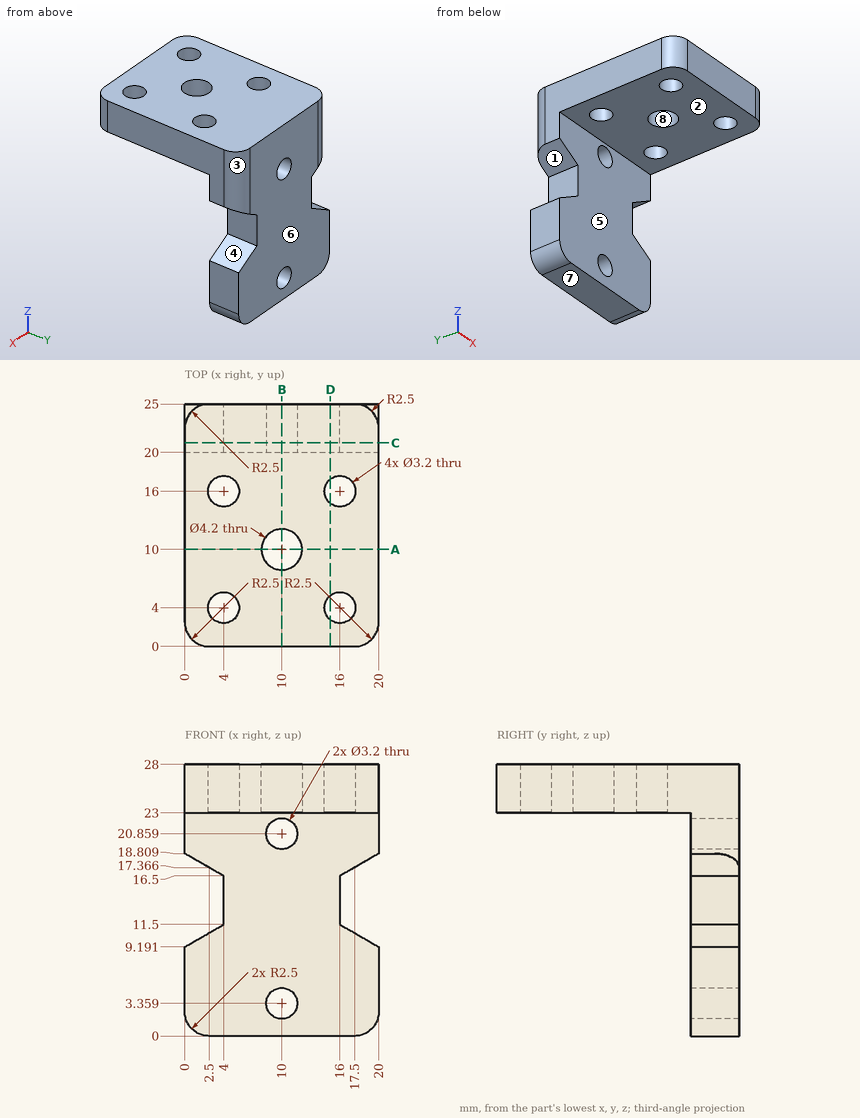
Can you work these out from the drawing? Everything is in mm from the part's minimum corner. A direction names the side the tool comes from. Coordinates: 2 decimals unless noted, no trailing zeros. Loops run counter-clockwise (first coordinate to the right, second up) from the corner with the lowest first, then second, coordinate; pieces in that order, holes last.
1. Imagine slicing it at D-D, the plane x = 15. Please give me the cut outline in (y, z), and give its area (3 significant figures).
2. For the marked faces 1, 2, 3 and 4, which set-ups out of +Z, -Z, +X, -X, +Y, -Y let a thin tool reach every point of the face, with its end or its side?
3. Imagine slicing it at A-A, the plane y = 10. Please give me the cut outline in (x, z).
4. Imagine slicing it at B-B, the plane x = 10. Please give me the cut outline in (y, z).
5. I need wall thicknesses on L1, parallel to Y at x = 4, z = 24.7; L2, parallel to Z at x = 10.5, y = 21.25; L3, parallel to Y at x = 1.75, z = 5.5. Which ranges of each line are inside material? Lowest first, please.
6. For P1, Ø3, axis at x = 14, y = 7, coming from the -Z side; P2, Ø2.5, axis at y = 23, z = 13, coming from the -X side; P3, Ø1.5, axis at y = 22, z = 13, coming from the +X side, each with a flat end and sliding along its axis, tell me the tip position at first contact or that it passes through.
7. Imagine slicing it at C-C, the plane y = 21. Please give me the cut outline in (x, z).
8. If we mould it in two halves opening along Y, with no side actions, what happens to the marked faces 5, 6, 7 and 8? For each: pulls with the +Y half, pulls with the -Y half, needs draft (parallel to the pull), parting line crosses it, or undercut.
Taken from the geometry:
1. outline: (0, 23) - (2.75, 23) - (2.75, 28) - (0, 28) - close; (5.25, 23) - (14.75, 23) - (14.75, 28) - (5.25, 28) - close; (17.25, 23) - (20, 23) - (20, 0) - (25, 0) - (25, 28) - (17.25, 28) - close
1. area: 215 mm2
2. face 1: -X, +Y, -Y
2. face 2: -Z, +X, -X, -Y
2. face 3: +Z, +X, +Y
2. face 4: +X, +Y, -Y
3. outline: (0, 23) - (7.9, 23) - (7.9, 28) - (0, 28) - close; (12.1, 23) - (20, 23) - (20, 28) - (12.1, 28) - close
4. outline: (0, 23) - (7.9, 23) - (7.9, 28) - (0, 28) - close; (12.1, 23) - (20, 23) - (20, 22.46) - (25, 22.46) - (25, 28) - (12.1, 28) - close; (20, 0) - (25, 0) - (25, 1.76) - (20, 1.76) - close; (20, 4.96) - (25, 4.96) - (25, 19.26) - (20, 19.26) - close
5. L1: y = 0 to 2.4, 5.6 to 14.4, 17.6 to 25
5. L2: z = 0 to 1.84, 4.88 to 19.34, 22.38 to 28
5. L3: y = 20 to 25
6. P1: stops at z = 23
6. P2: stops at x = 4
6. P3: stops at x = 16
7. outline: (0, 2.5) arc R2.5 ccw to (2.5, 0) - (17.5, 0) arc R2.5 ccw to (20, 2.5) - (20, 9.19) - (16, 11.5) - (16, 16.5) - (20, 18.81) - (20, 28) - (0, 28) - (0, 18.81) - (4, 16.5) - (4, 11.5) - (0, 9.19) - close; hole circle Ø3.2 at (10, 3.36); hole circle Ø3.2 at (10, 20.86)
8. face 5: pulls with the -Y half
8. face 6: pulls with the +Y half
8. face 7: needs draft
8. face 8: undercut
